```python
from build123d import *

# Parameters (mm, degrees)
EXTRUDE_2_DEPTH = 15


with BuildPart() as part:
    # 草图2 → 凸台-拉伸2 (new body)
    with BuildSketch(Plane.XY):
        Polygon((-359.835728953, 15), (40.164271047, 15), (40.164271047, 0), (-359.835728953, 0), (-370.899758445, -19.026698438), (-398.986364047, -2.810889132), (-381.486364047, 27.5), align=None)
        Polygon((-373.799917415, -9.77331612), (-391.073233535, 0.307980932), (-380.991936484, 17.581297051), (-363.718620364, 7.5), align=None, mode=Mode.SUBTRACT)
    extrude(amount=EXTRUDE_2_DEPTH)


solid = part.part
```
Geometry: final body of the model. Coordinates: model frame, mm. A direction names the side the tool comes from. Coordinates: 2 decimals unless noted, no trailing zeros. Order: outer loops, then holes, each group sorted by start corner. A loop starts at its lowest first (then second) coordinate and runs counter-clockwise, first axis right, second up. Notation, with made-up numbers: (50, -28) - (63, -28) arc R8 ccw to (63, -17) - close; hole circle Ø7 at (31.5, -38). An arc over 180 degrees is marked (long way). Write each question's results on one line, items separated by ' | '.
1) Pin query (flat end, axial travel): pin 1 (4.5 mm diameter, centred on x = -244, z = 9, fed in from -Y); pin 2 (2 mm diameter, centred on y = 12.5, z = 13.5, fed in from -X); pin 3 (4.5 mm diameter, centred on x = -185.5, z = 5.5, fed in from +Y). Return the tip coordinate at first contact, or that it passes through.
Results list:
pin 1: y = 0 | pin 2: x = -390.72 | pin 3: y = 15
2) Line query: line 1 (Y direction, x = -169, z = 9.75); line 2 (X direction, y = 3, z = 8); line 3 (Y direction, x = -379.5, z = 2.5). Output: solid intervals per line, ascending. Write a range as from..to.
Results list:
line 1: 0..15 | line 2: -395.63..-389.5, -366.34..40.16 | line 3: -14.06..-6.45, 16.71..26.35
3) Section A-A, the plane z = 6. Return loops of the section in (x, y).
Results list:
outline: (-398.99, -2.81) - (-370.9, -19.03) - (-359.84, 0) - (40.16, 0) - (40.16, 15) - (-359.84, 15) - (-381.49, 27.5) - close; hole (-391.07, 0.31) - (-373.8, -9.77) - (-363.72, 7.5) - (-380.99, 17.58) - close
4) Section B-B, the plane x = -8. Return loops of the section in (y, z), plus the area to 3 significant figures.
Results list:
outline: (0, 0) - (15, 0) - (15, 15) - (0, 15) - close | area: 225 mm^2
5) Set-up query: faces 5 (the flat face through (-157, 0, 7)), 6 (the flat face through (-368.69, -1.02, 7.4)), 7 (the flat face through (-390.36, 12.13, 7.4)). Return all of +Z, -Z, +X, -X, +Y, -Y with unobstructed straight access to the full face (end or side cutting, diameter ignored); none if empty.
Results list:
face 5: +Z, -Z, +X, -Y | face 6: +Z, -Z | face 7: +Z, -Z, -X, +Y
6) Section C-C, the plane y = -15. Return loops of the section in (x, z), plus the area to 3 significant figures.
Results list:
outline: (-377.87, 0) - (-368.56, 0) - (-368.56, 15) - (-377.87, 15) - close | area: 140 mm^2
7) Pull-direction query (X, two-part tool) for faces 1 (the flat face through (-163, 15, 7)), 2 (the flat face through (-370.813, 21.338, 7.395)), 3 (the flat face through (-384.75, -11.03, 7.4)), 4 (the flat face through (-386, 9, 7)); classes: pulls with the +X half, pulls with the -X half, needs draft (parallel to the pull), parting line crosses it, or undercut.
Results list:
face 1: needs draft | face 2: pulls with the +X half | face 3: pulls with the -X half | face 4: undercut
